```python
from build123d import *

# Parameters (mm, degrees)
SKETCH1_W           = 10
SKETCH1_H           = 30
SKETCH1_W_2         = 1
BOSS_EXTRUDE1_DEPTH = 1
BOSS_EXTRUDE4_START = 1
SKETCH1_3_W         = 34
SKETCH1_3_H         = 30
BOSS_EXTRUDE4_DEPTH = 6
BOSS_EXTRUDE5_START = 7
SKETCH1_4_W         = 10
SKETCH1_4_H         = 30
SKETCH1_4_W_2       = 12
BOSS_EXTRUDE5_DEPTH = 11
SKETCH3_W           = 8.5
SKETCH3_H           = 30
BOSS_EXTRUDE6_DEPTH = 4.5
CHAMFER1_SIZE       = 5
CHAMFER1_SIZE_2     = 3.501037691
SKETCH5_R           = 7.5
SKETCH5_R_2         = 4
CUT_EXTRUDE1_DEPTH  = 2.5
SKETCH5_3_R         = 4
CUT_EXTRUDE2_DEPTH  = 51.618672444
CUT_EXTRUDE4_START  = -27.5
SKETCH5_4_R         = 7.5
SKETCH5_4_R_2       = 4
CUT_EXTRUDE4_DEPTH  = 2.5
SKETCH6_R           = 2
CUT_EXTRUDE5_DEPTH  = 49.785243671


with BuildPart() as part:
    # Sketch1 → Boss-Extrude1 (new body)
    with BuildSketch(Plane(origin=(0, 0, 0), x_dir=(1, 0, 0), z_dir=(0, 1, 0))):
        with Locations((28, 15)):
            Rectangle(SKETCH1_W, SKETCH1_H)
        with Locations((33.5, 15)):
            Rectangle(SKETCH1_W_2, SKETCH1_H)
        with Locations((0.5, 15)):
            Rectangle(SKETCH1_W_2, SKETCH1_H)
        with Locations((6, 15)):
            Rectangle(SKETCH1_W, SKETCH1_H)
    extrude(amount=BOSS_EXTRUDE1_DEPTH)

    # Sketch1<3> → Boss-Extrude4 (add)
    with BuildSketch(Plane(origin=(0, 0, 0), x_dir=(1, 0, 0), z_dir=(0, 1, 0)).offset(BOSS_EXTRUDE4_START)):
        with Locations((17, 15)):
            Rectangle(SKETCH1_3_W, SKETCH1_3_H)
    extrude(amount=BOSS_EXTRUDE4_DEPTH)

    # Sketch1<4> → Boss-Extrude5 (add)
    with BuildSketch(Plane(origin=(0, 0, 0), x_dir=(1, 0, 0), z_dir=(0, 1, 0)).offset(BOSS_EXTRUDE5_START)):
        with Locations((6, 15)):
            Rectangle(SKETCH1_4_W, SKETCH1_4_H)
        with Locations((28, 15)):
            Rectangle(SKETCH1_4_W, SKETCH1_4_H)
        with Locations((17, 15)):
            Rectangle(SKETCH1_4_W_2, SKETCH1_4_H)
    extrude(amount=BOSS_EXTRUDE5_DEPTH)

    # Sketch3 → Boss-Extrude6 (add)
    with BuildSketch(Plane(origin=(0, 18, 0), x_dir=(1, 0, 0), z_dir=(0, 1, 0))):
        with Locations((21.25, 15)):
            Rectangle(SKETCH3_W, SKETCH3_H)
        with Locations((12.75, 15)):
            Rectangle(SKETCH3_W, SKETCH3_H)
    extrude(amount=BOSS_EXTRUDE6_DEPTH)

    # Chamfer1
    # the kernel refuses this chamfer: 5, 3.501037691 mm, written as the material it takes off along each edge
    with BuildSketch(Plane(origin=(25.5, 22.5, 12.912761151), x_dir=(0, -1, 0), z_dir=(0, 0, -1))) as chamfer1_piece_1_section:
        Polygon((CHAMFER1_SIZE, 0), (0, CHAMFER1_SIZE_2), (0, 0), align=None)
    chamfer1_piece_1 = extrude(amount=55.825522303, mode=Mode.PRIVATE)
    chamfer1_piece_1 = split(chamfer1_piece_1, bisect_by=Plane(origin=(25.5, 18, 12.912761151), z_dir=(0, 1, 0)), keep=Keep.TOP, mode=Mode.PRIVATE)
    add(chamfer1_piece_1, mode=Mode.SUBTRACT)
    with BuildSketch(Plane(origin=(8.5, 22.5, -42.912761151), x_dir=(0, -1, 0), z_dir=(0, 0, 1))) as chamfer1_piece_2_section:
        Polygon((CHAMFER1_SIZE, 0), (0, CHAMFER1_SIZE_2), (0, 0), align=None)
    chamfer1_piece_2 = extrude(amount=55.825522303, mode=Mode.PRIVATE)
    chamfer1_piece_2 = split(chamfer1_piece_2, bisect_by=Plane(origin=(8.5, 18, -42.912761151), z_dir=(0, 1, 0)), keep=Keep.TOP, mode=Mode.PRIVATE)
    add(chamfer1_piece_2, mode=Mode.SUBTRACT)

    # Sketch5 → Cut-Extrude1 (cut)
    # profile 1 of 2: a face of its own
    with BuildSketch(Plane.XY):
        with Locations((17, 11.5)):
            Circle(SKETCH5_R)
        with Locations((17, 11.5)):
            Circle(SKETCH5_R_2, mode=Mode.SUBTRACT)
    # profile 2 of 2: a face of its own
    with BuildSketch(Plane.XY):
        with Locations((17, 11.5)):
            Circle(SKETCH5_R_2)
    extrude(amount=-CUT_EXTRUDE1_DEPTH, mode=Mode.SUBTRACT)

    # Sketch5<3> → Cut-Extrude2 (cut, through all)
    with BuildSketch(Plane.XY):
        with Locations((17, 11.5)):
            Circle(SKETCH5_3_R)
    extrude(amount=-CUT_EXTRUDE2_DEPTH, mode=Mode.SUBTRACT)

    # Sketch5<4> → Cut-Extrude4 (cut)
    # profile 1 of 2: a face of its own
    with BuildSketch(Plane.XY.offset(CUT_EXTRUDE4_START)):
        with Locations((17, 11.5)):
            Circle(SKETCH5_4_R)
        with Locations((17, 11.5)):
            Circle(SKETCH5_4_R_2, mode=Mode.SUBTRACT)
    # profile 2 of 2: a face of its own
    with BuildSketch(Plane.XY.offset(CUT_EXTRUDE4_START)):
        with Locations((17, 11.5)):
            Circle(SKETCH5_4_R_2)
    extrude(amount=-CUT_EXTRUDE4_DEPTH, mode=Mode.SUBTRACT)

    # Sketch6 → Cut-Extrude5 (cut, through all)
    with BuildSketch(Plane(origin=(0, 18, 0), x_dir=(1, 0, 0), z_dir=(0, 1, 0))):
        with Locations(Location((29.5, 24.5, 0), (0, 0, 270))):
            Circle(SKETCH6_R)
        with Locations(Location((29.5, 5.5, 0), (0, 0, 270))):
            Circle(SKETCH6_R)
        with Locations(Location((4.5, 24.5, 0), (0, 0, 90))):
            Circle(SKETCH6_R)
        with Locations(Location((4.5, 5.5, 0), (0, 0, 90))):
            Circle(SKETCH6_R)
    extrude(amount=-CUT_EXTRUDE5_DEPTH, mode=Mode.SUBTRACT)


solid = part.part
```
Geometry: final body of the model. Coordinates: model frame, mm. A direction names the side the tool comes from. Coordinates: 2 decimals unless noted, no trailing zeros. Order: outer loops, then holes, each group sorted by start corner. A loop starts at its lowest first (then second) coordinate and runs counter-clockwise, first axis right, second up. Notation, with made-up numbers: (4.25, 16.5) - (60.25, 16.5) arc R24 ccw to (60.25, 28.5) - close; hole circle Ø11 at (4.25, 12). An arc over 180 degrees is marked (long way). Write each question's results on one line, items separated by ' | '.
1) Section D-D, the plane z = -21. Return loops of the section in (x, y), plus the area to 3 significant figures.
Results list:
outline: (0, 0) - (11, 0) - (11, 1) - (23, 1) - (23, 0) - (34, 0) - (34, 7) - (33, 7) - (33, 18) - (25.15, 18) - (22, 22.5) - (12, 22.5) - (8.85, 18) - (1, 18) - (1, 7) - (0, 7) - close; hole circle Ø8 at (17, 11.5) | area: 587 mm^2
2) Line query: line 1 (Z direction, x = 4.5, y = 5); line 2 (X direction, y = 9.75, z = -5.5); line 3 (X direction, y = 6, z = -4). Output: solid intervals per line, ascending. Write a range as from..to.
Results list:
line 1: -30..-26.5, -22.5..-7.5, -3.5..0 | line 2: 1..2.5, 6.5..13.4, 20.6..27.5, 31.5..33 | line 3: 0..3.18, 5.82..28.18, 30.82..34
3) Pull-direction query (Z, two-part tool) for faces 1 (the flat face through (20, 8, -2.5)), 2 (the cylindrical face through (27.548, 9.126, -5.934)), 3 (the flat face through (0, 3, -15)); classes: pulls with the +Z half, pulls with the -Z half, needs draft (parallel to the pull), parting line crosses it, or undercut.
Results list:
face 1: pulls with the +Z half | face 2: undercut | face 3: needs draft
4) Section B-B, the plane x = 4.5. Return loops of the section in (y, z).
Results list:
outline: (0, -30) - (18, -30) - (18, -26.5) - (0, -26.5) - close; (0, -22.5) - (18, -22.5) - (18, -7.5) - (0, -7.5) - close; (0, -3.5) - (18, -3.5) - (18, 0) - (0, 0) - close
5) Section C-C, the plane y = 11.5. Return loops of the section in (x, z).
Results list:
outline: (1, -30) - (9.5, -30) - (9.5, -27.5) - (13, -27.5) - (13, -2.5) - (9.5, -2.5) - (9.5, 0) - (1, 0) - close; (21, -27.5) - (24.5, -27.5) - (24.5, -30) - (33, -30) - (33, 0) - (24.5, 0) - (24.5, -2.5) - (21, -2.5) - close; hole circle Ø4 at (4.5, -24.5); hole circle Ø4 at (4.5, -5.5); hole circle Ø4 at (29.5, -24.5); hole circle Ø4 at (29.5, -5.5)
6) Pin query (flat end, axial travel): pin 1 (10 mm diameter, centred on x = 30.5, z = -20, fed in from -Y); pin 2 (9.5 mm diameter, centred on x = 17.5, z = -13.5, fed in from -Y); pin 3 (13 mm diameter, centred on x = 17, y = 11.5, fed in from +Z); pin 4 (2 mm diameter, centred on x = 21.5, y = 10, fed in from -Z). Return the tip coordinate at first contact, or that it passes through.
Results list:
pin 1: y = 0 | pin 2: y = 1 | pin 3: z = -2.5 | pin 4: z = -27.5
7) Section A-A, the plane z = -5.5. Return loops of the section in (x, y).
Results list:
outline: (0, 0) - (2.5, 0) - (2.5, 18) - (1, 18) - (1, 7) - (0, 7) - close; (6.5, 0) - (11, 0) - (11, 1) - (23, 1) - (23, 0) - (27.5, 0) - (27.5, 18) - (25.15, 18) - (22, 22.5) - (12, 22.5) - (8.85, 18) - (6.5, 18) - close; (31.5, 0) - (34, 0) - (34, 7) - (33, 7) - (33, 18) - (31.5, 18) - close; hole circle Ø8 at (17, 11.5)
8) Set-up query: faces 4 (the cylindrical face through (11, 7, -29)), 5 (the cylindrical face through (5.7, 9.1, -3.9)), 6 (the flat face through (29, 18, -15)), 7 (the flat face through (5, 18, -15)), 8 (the flat face through (23, 0.5, -14.8)). Return all of +Z, -Z, +X, -X, +Y, -Y with unobstructed straight access to the full face (end or side cutting, diameter ignored); none if empty.
Results list:
face 4: -Z | face 5: +Y, -Y | face 6: +Z, -Z, +X, +Y | face 7: +Z, -Z, -X, +Y | face 8: +Z, -Z, -Y
